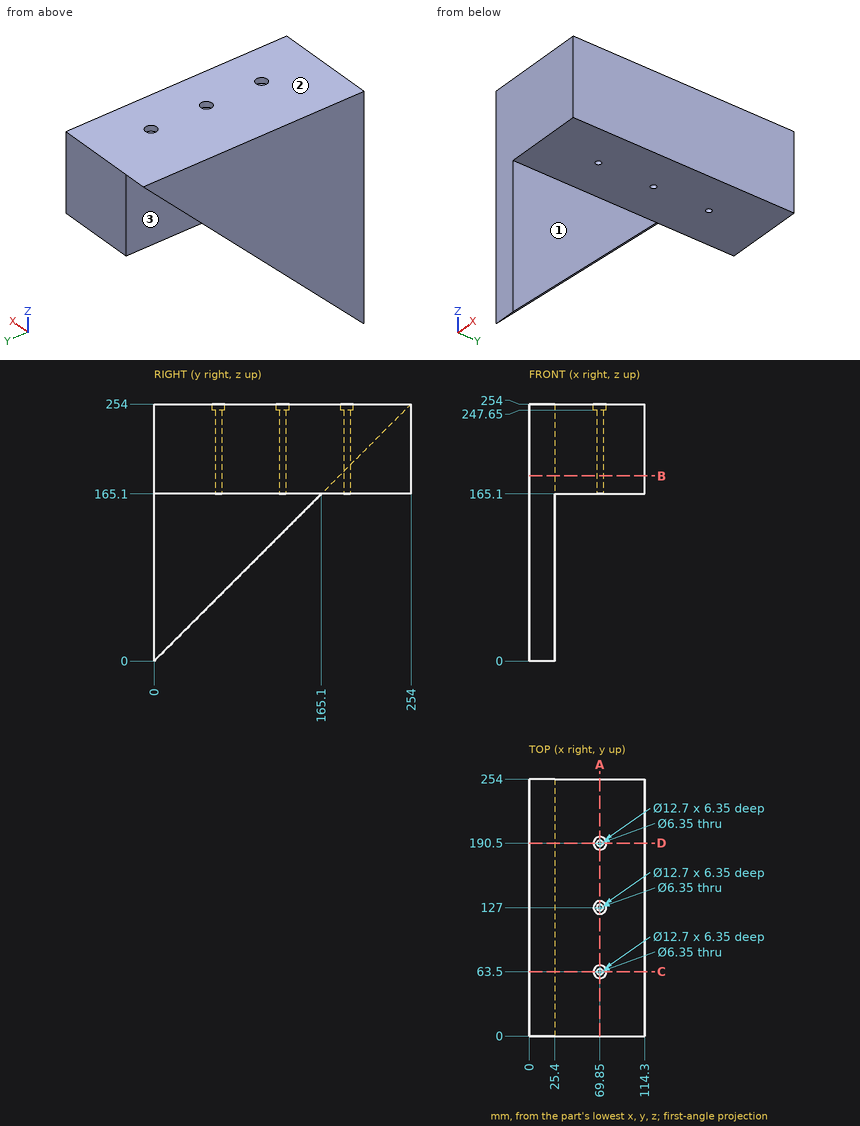
Geometry: see drawing. Coordinates: mm, zero at the bounding-box minimum. A direction names the side the tool comes from. Round coordinates to 2 decimals unless told otherwise and drop trailing zeros. Loops run counter-clockwise (first coordinate to the right, second up) from the corner with the lowest first, then second, coordinate; pieces in that order, holes last. Notation, with made-up numbers: (8.25, 42.25) - (61.25, 42.25) arc R31 cw to (61.25, 81.25) - close; hole circle Ø5 at (-39.5, 32.25). An arc over 180 degrees is marked (long way). One line per item, written item: value. Start each with the question number.
(1) Section A-A, the plane x = 69.85. Return loops of the section in (y, z) (3 decimals), plus the area to 3 significant figures.
(2) Section D-D, the plane y = 190.5. Return loops of the section in (x, z) (3 decimals).
(3) Section C-C, the plane y = 63.5. Return loops of the section in (x, z) (3 decimals).
(4) Ray query, line 1 (Y direction, x = 69, z = 249); line 2 (X direction, y = 190, z = 252); line 3 (Y direction, x = 69.85, z = 187) (3 decimals). Return the intervals inside material, ascending. Write a range as [from, to].
(5) Contact query for flat-ended pins moving along their axis: P1, Ø10, axis at x = 69, y = 190, coming from the +Z side; P2, Ø8.5, axis at x = 69.85, y = 127, coming from the -Z side. Output: stop coordinate, or through.
(6) Section B-B, the plane z = 183. Return loops of the section in (x, y) (3 decimals).
(7) Access query for the marked faces 1, 2 and 3. Directions: +Z, -Z, +X, -X, +Y, -Y. A direction counts if a zero-diameter tool reaches every point of the face in a straight line with its end or side. Return the directions, or none.
Results below:
1. outline: (0, 165.1) - (60.325, 165.1) - (60.325, 247.65) - (57.15, 247.65) - (57.15, 254) - (0, 254) - close; (66.675, 165.1) - (123.825, 165.1) - (123.825, 247.65) - (120.65, 247.65) - (120.65, 254) - (69.85, 254) - (69.85, 247.65) - (66.675, 247.65) - close; (130.175, 165.1) - (187.325, 165.1) - (187.325, 247.65) - (184.15, 247.65) - (184.15, 254) - (133.35, 254) - (133.35, 247.65) - (130.175, 247.65) - close; (193.675, 165.1) - (254, 165.1) - (254, 254) - (196.85, 254) - (196.85, 247.65) - (193.675, 247.65) - close
1. area: 20,800 mm^2
2. outline: (0, 190.5) - (25.4, 190.5) - (25.4, 165.1) - (66.675, 165.1) - (66.675, 247.65) - (63.5, 247.65) - (63.5, 254) - (0, 254) - close; (73.025, 165.1) - (114.3, 165.1) - (114.3, 254) - (76.2, 254) - (76.2, 247.65) - (73.025, 247.65) - close
3. outline: (0, 63.5) - (25.4, 63.5) - (25.4, 165.1) - (66.675, 165.1) - (66.675, 247.65) - (63.5, 247.65) - (63.5, 254) - (0, 254) - close; (73.025, 165.1) - (114.3, 165.1) - (114.3, 254) - (76.2, 254) - (76.2, 247.65) - (73.025, 247.65) - close
4. line 1: [0, 57.21], [69.79, 120.71], [133.29, 184.21], [196.79, 254]
4. line 2: [0, 63.52], [76.18, 114.3]
4. line 3: [0, 60.325], [66.675, 123.825], [130.175, 187.325], [193.675, 254]
5. P1: z = 247.65
5. P2: z = 165.1
6. outline: (0, 0) - (114.3, 0) - (114.3, 254) - (25.4, 254) - (25.4, 183) - (0, 183) - close; hole circle Ø6.35 at (69.85, 63.5); hole circle Ø6.35 at (69.85, 127); hole circle Ø6.35 at (69.85, 190.5)
7. face 1: -Z, +X, +Y, -Y
7. face 2: +Z, +X, -X, +Y, -Y
7. face 3: -Z, -X, +Y
